Autodesk Inventor part; units mm, degrees
ref_plane "YZ Plane" through (0, 0, 0) normal (1, 0, 0) x (0, 1, 0)
ref_plane "XZ Plane" through (0, 0, 0) normal (0, 1, 0) x (-1, 0, 0)
ref_plane "XY Plane" through (0, 0, 0) normal (0, 0, 1) x (1, 0, 0)
sketch "スケッチ1" plane through (0, 0, 0) normal (0, 0, 1) x (1, 0, 0)
  line L0 (-7, -29) -> (-7, -27)
  arc A0 (-6, -26) -> (-7, -27) centre (-6, -27) ccw
  line L1 (-6, -26) -> (-4.1307, -26)
  arc A1 (-3.1588, -27.2353) -> (-4.1307, -26) centre (-4.1307, -27) ccw
  arc A2 (-3.1588, -27.2353) -> (-3.1588, -28.7647) centre (0, -28) ccw
  arc A3 (-4.1307, -30) -> (-3.1588, -28.7647) centre (-4.1307, -29) ccw
  line L2 (-4.1307, -30) -> (-6, -30)
  arc A4 (-7, -29) -> (-6, -30) centre (-6, -29) ccw
  arc A5 (-6.5, -22.1534) -> (-5.5, -24) centre (-6, -23.0767) ccw
  line L3 (-6.5, -21) -> (-6.5, -22.1534)
  line L4 (-9, -21) -> (-6.5, -21)
  line L5 (-9, -35) -> (-9, -21)
  line L6 (-6.5, -35) -> (-9, -35)
  line L7 (-6.5, -33.8466) -> (-6.5, -35)
  arc A6 (-5.5, -32) -> (-6.5, -33.8466) centre (-6, -32.9233) ccw
  line L8 (-3.5, -32) -> (-5.5, -32)
  line L9 (0.6267, -31.189) -> (-3.5, -32)
  arc A7 (0.6267, -31.189) -> (0.6267, -24.811) centre (0, -28) ccw
  line L10 (-3.5, -24) -> (0.6267, -24.811)
  line L11 (-5.5, -24) -> (-3.5, -24)
  circle A8 centre (0, -28) radius 1.25
  line L12 (-7, -15) -> (-7, -13)
  arc A9 (-6, -12) -> (-7, -13) centre (-6, -13) ccw
  line L13 (-6, -12) -> (-4.1307, -12)
  arc A10 (-3.1588, -13.2353) -> (-4.1307, -12) centre (-4.1307, -13) ccw
  arc A11 (-3.1588, -13.2353) -> (-3.1588, -14.7647) centre (0, -14) ccw
  arc A12 (-4.1307, -16) -> (-3.1588, -14.7647) centre (-4.1307, -15) ccw
  line L14 (-4.1307, -16) -> (-6, -16)
  arc A13 (-7, -15) -> (-6, -16) centre (-6, -15) ccw
  arc A14 (-6.5, -8.1534) -> (-5.5, -10) centre (-6, -9.0767) ccw
  line L15 (-6.5, -7) -> (-6.5, -8.1534)
  line L16 (-9, -7) -> (-6.5, -7)
  line L17 (-9, -21) -> (-9, -7)
  line L18 (-6.5, -21) -> (-9, -21)
  line L19 (-6.5, -19.8466) -> (-6.5, -21)
  arc A15 (-5.5, -18) -> (-6.5, -19.8466) centre (-6, -18.9233) ccw
  line L20 (-3.5, -18) -> (-5.5, -18)
  line L21 (0.6267, -17.189) -> (-3.5, -18)
  arc A16 (0.6267, -17.189) -> (0.6267, -10.811) centre (0, -14) ccw
  line L22 (-3.5, -10) -> (0.6267, -10.811)
  line L23 (-5.5, -10) -> (-3.5, -10)
  circle A17 centre (0, -14) radius 1.25
  line L24 (-7, -1) -> (-7, 1)
  arc A18 (-6, 2) -> (-7, 1) centre (-6, 1) ccw
  line L25 (-6, 2) -> (-4.1307, 2)
  arc A19 (-3.1588, 0.7647) -> (-4.1307, 2) centre (-4.1307, 1) ccw
  arc A20 (-3.1588, 0.7647) -> (-3.1588, -0.7647) centre (0, 0) ccw
  arc A21 (-4.1307, -2) -> (-3.1588, -0.7647) centre (-4.1307, -1) ccw
  line L26 (-4.1307, -2) -> (-6, -2)
  arc A22 (-7, -1) -> (-6, -2) centre (-6, -1) ccw
  arc A23 (-6.5, 5.8466) -> (-5.5, 4) centre (-6, 4.9233) ccw
  line L27 (-6.5, 7) -> (-6.5, 5.8466)
  line L28 (-9, 7) -> (-6.5, 7)
  line L29 (-9, -7) -> (-9, 7)
  line L30 (-6.5, -7) -> (-9, -7)
  line L31 (-6.5, -5.8466) -> (-6.5, -7)
  arc A24 (-5.5, -4) -> (-6.5, -5.8466) centre (-6, -4.9233) ccw
  line L32 (-3.5, -4) -> (-5.5, -4)
  line L33 (0.6267, -3.189) -> (-3.5, -4)
  arc A25 (0.6267, -3.189) -> (0.6267, 3.189) centre (0, 0) ccw
  line L34 (-3.5, 4) -> (0.6267, 3.189)
  line L35 (-5.5, 4) -> (-3.5, 4)
  circle A26 centre (0, 0) radius 1.25
extrude "押し出し1" add sketch "スケッチ1" along normal blind 3
properties part number "アームユニット底板締結パーツ3t用" material "アルミニウム 2014-T4"
Geometry: final body of the model. Coordinates: model frame, mm. A direction names the side the tool comes from. Coordinates: 2 decimals unless noted, no trailing zeros. Loops run counter-clockwise (first coordinate to the right, second up) from the corner with the lowest first, then second, coordinate; pieces in that order, holes last. Notation, with made-up numbers: (62.25, -35) -> (117.25, -35) arc R12 cw to (117.25, -14) -> close; hole circle Ø4 at (19.5, 57.5). An arc over 180 degrees is marked (long way). Use a Markdown table: item, result. Add a question column.
(1) Line query: line 1 along Y through (x, z) = (-4.5, 2.25); line 2 along Y through (x, z) = (0, 2.3); line 3 along X through (y, z) = (-13, 0.85). Output: solid intervals per line, ascending.
(2) Section query C-C, the plane z = 1.35. State how many separate pieces and enclosed holes the cut face has, plus the area to 3 significant figures.
(3) Access query for faces 1 (the flat face through (-1.41, -3.59, 1.48)), 2 (the cylindrical face through (-6.715, -12.301, 1.479)). Directions: +Z, -Z, +X, -X, +Y, -Y. A direction counts if a zero-diameter tool reaches every point of the face in a straight line with its end or side. Return the directions, or none.
(4) Section query B-B, the plane x = -4.5. Return loops of the section in (y, z), plus the area to 3 significant figures.
(5) Pin query (flat end, axial travel): pin 1 Ø0.9 at (x, z) = (-4.5, 1) entering from -Y; pin 2 Ø1.5 at (x, z) = (-5.5, 1.5) entering from +Y; pin 3 Ø1.2 at (y, z) = (-21, 1.5) entering from +X. Return the tip coordinate at first contact, or that it passes through.
(6) Section query A-A, the plane y = 0. Return loops of the section in (x, z).
(7) Mould query, pull axis Y, two halves, no side actions, for faces 3 (the flat face through (-3, -12, 3)), 4 (the cylindrical face through (-3.34, -1.61, 1.48)). Classes: pulls with the +Y half, pulls with the -Y half, needs draft (parallel to the pull), parting line crosses it, or undercut.
(8) Section query D-D, the plane y = -20.5. Return loops of the section in (x, z), plus the area to 3 significant figures.
Answer:
| question | item | result |
|---|---|---|
| 1 | line 1 | y = -32 to -30, -26 to -24, -18 to -16, -12 to -10, -4 to -2, 2 to 4 |
| 1 | line 2 | y = -31.31 to -29.25, -26.75 to -24.69, -17.31 to -15.25, -12.75 to -10.69, -3.31 to -1.25, 1.25 to 3.31 |
| 1 | line 3 | x = -9 to -7, -3.13 to -0.75, 0.75 to 3.09 |
| 2 | separate pieces | 1 |
| 2 | enclosed holes | 6 |
| 2 | area | 241 mm^2 |
| 3 | face 1 | +Z, -Z, +X |
| 3 | face 2 | +Z, -Z |
| 4 | outline | (-32, 0) -> (-30, 0) -> (-30, 3) -> (-32, 3) -> close; (-26, 0) -> (-24, 0) -> (-24, 3) -> (-26, 3) -> close; (-18, 0) -> (-16, 0) -> (-16, 3) -> (-18, 3) -> close; (-12, 0) -> (-10, 0) -> (-10, 3) -> (-12, 3) -> close; (-4, 0) -> (-2, 0) -> (-2, 3) -> (-4, 3) -> close; (2, 0) -> (4, 0) -> (4, 3) -> (2, 3) -> close |
| 4 | area | 36.0 mm^2 |
| 5 | pin 1 | stops at y = -32 |
| 5 | pin 2 | stops at y = 4 |
| 5 | pin 3 | stops at x = -6.5 |
| 6 | outline | (-9, 0) -> (-7, 0) -> (-7, 3) -> (-9, 3) -> close; (-3.25, 0) -> (-1.25, 0) -> (-1.25, 3) -> (-3.25, 3) -> close; (1.25, 0) -> (3.25, 0) -> (3.25, 3) -> (1.25, 3) -> close |
| 7 | face 3 | needs draft |
| 7 | face 4 | undercut |
| 8 | outline | (-9, 0) -> (-6.5, 0) -> (-6.5, 3) -> (-9, 3) -> close |
| 8 | area | 7.50 mm^2 |
